Could you check a few things on this model? Use its own coordinates, in mm. A direction names the side the tool comes from. Give positions to 0.01 mm unless a question says otherwise; leave off trailing zeros. Order: outer loops, then holes, each group sorted by start corner. A loop starts at its lowest first (then second) coordinate and runs counter-clockwise, first axis right, second up.
from build123d import *

# Parameters (mm, degrees)
SKETCH1_R           = 10.125
BOSS_EXTRUDE1_DEPTH = 10
SKETCH2_R           = 10.125
BOSS_EXTRUDE2_DEPTH = 30


with BuildPart() as part:
    # Sketch1 → Boss-Extrude1 (new body)
    with BuildSketch(Plane(origin=(0, 0, 0), x_dir=(1, 0, 0), z_dir=(0, 1, 0))):
        Circle(SKETCH1_R)
        with BuildLine():
            Line((9.3566828, 0.79375), (5.365749064, 7.70625))
            ThreePointArc((5.365749064, 7.70625), (4.784683736, 8.287315329), (3.990933736, 8.5))
            Line((3.990933736, 8.5), (-3.990933736, 8.5))
            ThreePointArc((-3.990933736, 8.5), (-4.784683736, 8.287315329), (-5.365749064, 7.70625))
            Line((-5.365749064, 7.70625), (-9.3566828, 0.79375))
            ThreePointArc((-9.3566828, 0.79375), (-9.569367472, 0), (-9.3566828, -0.79375))
            Line((-9.3566828, -0.79375), (-5.365749064, -7.70625))
            ThreePointArc((-5.365749064, -7.70625), (-4.784683736, -8.287315329), (-3.990933736, -8.5))
            Line((-3.990933736, -8.5), (3.990933736, -8.5))
            ThreePointArc((3.990933736, -8.5), (4.784683736, -8.287315329), (5.365749064, -7.70625))
            Line((5.365749064, -7.70625), (9.3566828, -0.79375))
            ThreePointArc((9.3566828, -0.79375), (9.569367472, 0), (9.3566828, 0.79375))
        make_face(mode=Mode.SUBTRACT)
    extrude(amount=BOSS_EXTRUDE1_DEPTH)

    # Sketch2 → Boss-Extrude2 (add)
    with BuildSketch(Plane(origin=(0, 10, 0), x_dir=(1, 0, 0), z_dir=(0, 1, 0))):
        Circle(SKETCH2_R)
    extrude(amount=BOSS_EXTRUDE2_DEPTH)


solid = part.part
Item 1: For faces 4 (the flat face through (0, 40, 0)), 5 (the cylindrical face through (-4.775, 4.93, -8.293)), which set-ups out of +Z, -Z, +X, -X, +Y, -Y let a thin tool reach every point of the face, with its end or its side?
Findings:
face 4: +Z, -Z, +X, -X, +Y
face 5: -Y
Item 2: Please list where these lines run through material, in increasing order: line 1 along Y through (x, z) = (1.5, -6.5); line 2 along Z through (x, y) = (-5.5, 14); line 3 along Z through (x, y) = (-7, 6.5).
Findings:
line 1: y = 10 to 40
line 2: z = -8.5 to 8.5
line 3: z = -7.32 to -4.88, 4.88 to 7.32
Item 3: Imagine slicing it at C-C on y = 17. List the corners of the cut face in (x, z) for me (3 decimals), then the cut area to 3 significant figures.
Findings:
outline: circle Ø20.25 at (0, 0)
area: 322 mm2
Item 4: Imagine slicing it at B-B on x = 0. List the corners of the cut face in (y, z) for me (3 decimals), then the cut area to 3 significant figures.
Findings:
outline: (0, -10.125) - (40, -10.125) - (40, 10.125) - (0, 10.125) - (0, 8.5) - (10, 8.5) - (10, -8.5) - (0, -8.5) - close
area: 640 mm2
Item 5: For pin 1 (8 mm diameter, centred on x = 7, y = 11, fed in from -Z); pin 2 (1 mm diameter, centred on x = -4, y = 21, fed in from +Z); pin 3 (1 mm diameter, centred on y = 12, z = -2, fed in from +X), each with a flat end and sliding along its axis, tell me the tip position at first contact or that it passes through.
Findings:
pin 1: stops at z = -9.67
pin 2: stops at z = 9.5
pin 3: stops at x = 10.01
Item 6: Imagine slicing it at A-A on z = 0. List the corners of the cut face in (x, y) for me (3 decimals).
Findings:
outline: (-10.125, 0) - (-9.569, 0) - (-9.569, 10) - (9.569, 10) - (9.569, 0) - (10.125, 0) - (10.125, 40) - (-10.125, 40) - close
Item 7: We'd pull the mould along Z, two halves only. Please class faces 1 (the cylindrical face through (5.44, 19.72, -8.54)), 2 (the cylindrical face through (9.57, 4.93, 0.01)), 3 (the flat face through (7.5, 0, -4.5)): +Z half, -Z half, draft (parallel to the pull), parting line (faces both ways), or undercut.
Findings:
face 1: parting line
face 2: undercut
face 3: draft
